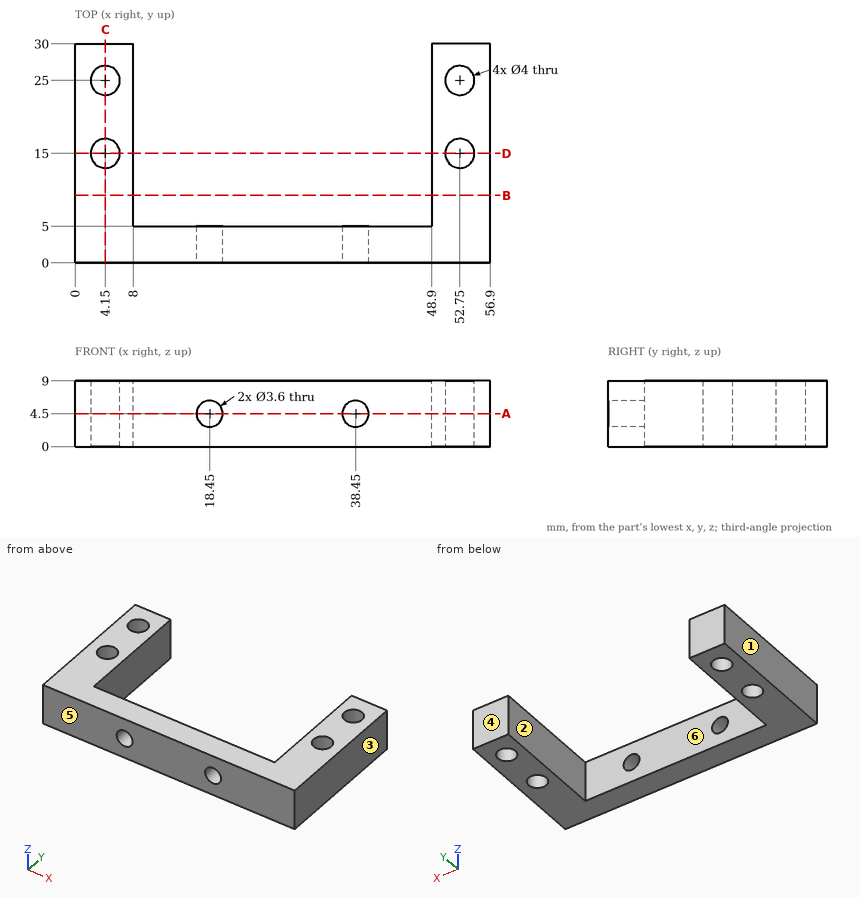
Check sheet for the drawn part. Datum: minimum x, y, z corner. Units: mm. A direction names the side the tool comes from. Round coordinates to 2 decimals unless told otherwise and drop trailing zeros. Write each loop counter-clockwise with the first axis right and the second up, starting at its lowest first coordinate (ties: lowest second). Pieces come first, ordered by that corner, then holes. Notation, with made-up numbers: (-31, 80) -> (-25, 80) arc R23 cw to (-25, 119) -> close; hole circle Ø7 at (-35, 5). An arc over 180 degrees is marked (long way). One line per item, written item: value. Start each with the question number.
(1) Cross-section at A-A, the plane z = 4.5. Record the cut outline in (x, y).
(2) Cross-section at B-B, the plane y = 9.25. Record the cut outline in (x, z).
(3) Cross-section at C-C, the plane x = 4.15. Record the cut outline in (y, z), and give its area (3 significant figures).
(4) Go/stop test with flat-tipped pins: pin 1 Ø4.5 at (x, z) = (27.5, 3.5) entering from +Y; pin 2 Ø3.5 at (x, y) = (4.15, 15) entering from +Z. Record where each tip stops, or that it passes through.
(5) Cross-section at D-D, the plane y = 15. Record the cut outline in (x, z).
(6) Draft check along X on the marked faces 1, 2, 3 and 4. Enter one of: +X half, -X half, draft (parallel to the pull), parting line (faces both ways), or undercut.
(7) Access from +Z, -Z, +X, -X, +Y, -Y to the whole of each face (thin tool, end or side, straight path). Record for the marked faces 5 and 6.
(8) Scan lines: line 1 (Y direction, x = 4.15, z = 5.25); line 2 (X direction, y = 10, z = 7); line 3 (Z direction, x = 18.45, y = 3.1). Record each from-to range of solid material in increasing order. Write a range as [from, to].
Answer:
1. outline: (0, 0) -> (16.65, 0) -> (16.65, 5) -> (8, 5) -> (8, 30) -> (0, 30) -> close; (20.25, 0) -> (36.65, 0) -> (36.65, 5) -> (20.25, 5) -> close; (40.25, 0) -> (56.9, 0) -> (56.9, 30) -> (48.9, 30) -> (48.9, 5) -> (40.25, 5) -> close; hole circle Ø4 at (4.15, 15); hole circle Ø4 at (4.15, 25); hole circle Ø4 at (52.75, 15); hole circle Ø4 at (52.75, 25)
2. outline: (0, 0) -> (8, 0) -> (8, 9) -> (0, 9) -> close; (48.9, 0) -> (56.9, 0) -> (56.9, 9) -> (48.9, 9) -> close
3. outline: (0, 0) -> (13, 0) -> (13, 9) -> (0, 9) -> close; (17, 0) -> (23, 0) -> (23, 9) -> (17, 9) -> close; (27, 0) -> (30, 0) -> (30, 9) -> (27, 9) -> close
3. area: 198 mm²
4. pin 1: y = 5
4. pin 2: through
5. outline: (0, 0) -> (2.15, 0) -> (2.15, 9) -> (0, 9) -> close; (6.15, 0) -> (8, 0) -> (8, 9) -> (6.15, 9) -> close; (48.9, 0) -> (50.75, 0) -> (50.75, 9) -> (48.9, 9) -> close; (54.75, 0) -> (56.9, 0) -> (56.9, 9) -> (54.75, 9) -> close
6. face 1: -X half
6. face 2: undercut
6. face 3: +X half
6. face 4: draft
7. face 5: +Z, -Z, +X, -X, -Y
7. face 6: +Z, -Z, +Y
8. line 1: [0, 13], [17, 23], [27, 30]
8. line 2: [0, 8], [48.9, 56.9]
8. line 3: [0, 2.7], [6.3, 9]
